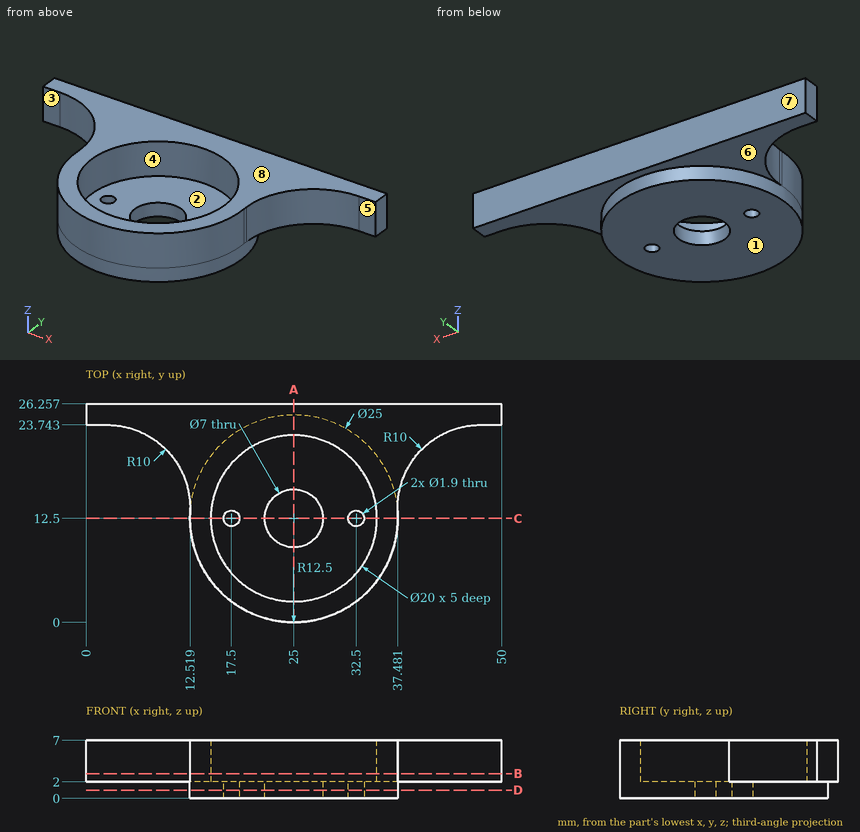
Job drawing, mm, ordinate dimensions from the low corner. One solid piece. A direction names the side the tool comes from. Round coordinates to 2 decimals unless told otherwise and drop trailing zeros. Order: outer loops, then holes, each group sorted by start corner. A loop starts at its lowest first (then second) coordinate and runs counter-clockwise, first axis right, second up. Notation, with made-up numbers: (84.25, -31.5) -> (134.25, -31.5) arc R19 cw to (134.25, -15.5) -> close; hole circle Ø4 at (84, 44.25). An arc over 180 degrees is marked (long way). Write item = value, one per line.
(1) Cut at A-A (x = 25). Write the cut outline in (y, z).
Answers follow:
outline = (0, 0) -> (9, 0) -> (9, 2) -> (2.5, 2) -> (2.5, 7) -> (0, 7) -> close; (16, 0) -> (25, 0) -> (25, 2) -> (26.26, 2) -> (26.26, 7) -> (22.5, 7) -> (22.5, 2) -> (16, 2) -> close
(2) Cut at C-C (y = 12.5). Write the cut outline in (x, z), plus the area to 3 significant figures.
Answers follow:
outline = (12.5, 0) -> (16.55, 0) -> (16.55, 2) -> (15, 2) -> (15, 7) -> (12.5, 7) -> close; (18.45, 0) -> (21.5, 0) -> (21.5, 2) -> (18.45, 2) -> close; (28.5, 0) -> (31.55, 0) -> (31.55, 2) -> (28.5, 2) -> close; (33.45, 0) -> (37.5, 0) -> (37.5, 7) -> (35, 7) -> (35, 2) -> (33.45, 2) -> close
area = 53.4 mm²
(3) Cut at B-B (z = 3). Write the cut outline in (x, y).
Answers follow:
outline = (0, 23.74) -> (2.52, 23.74) arc R10 cw to (12.52, 13.74) -> (12.52, 13.19) arc R12.5 ccw (long way) to (37.48, 13.19) -> (37.48, 13.74) arc R10 cw to (47.48, 23.74) -> (50, 23.74) -> (50, 26.26) -> (0, 26.26) -> close; hole circle Ø20 at (25, 12.5)
(4) Drill centre lines: L1, parallel to Y at x = 32.5, z = 1.4; L2, parallel to Y at x = 25, z = 3.1; L3, parallel to Z at x = 25, y = 5.25. Where is each one in solid material? Low to high.
Answers follow:
L1 = 2.5 to 11.55, 13.45 to 22.5
L2 = 0 to 2.5, 22.5 to 26.26
L3 = 0 to 2
(5) Cut at D-D (z = 1). Write the cut outline in (x, y).
Answers follow:
outline = circle Ø25 at (25, 12.5); hole circle Ø1.9 at (17.5, 12.5); hole circle Ø7 at (25, 12.5); hole circle Ø1.9 at (32.5, 12.5)
(6) Pull direction Y, two halves, no side cores. Call the marked faces 1, 2 and 3: +Y half, -Y half, draft (parallel to the pull), parting line (faces both ways), or undercut.
Answers follow:
face_1 = draft
face_2 = undercut
face_3 = -Y half
(7) 3-axis set-ups, long thin cutter, end or side, ignore diameter. For the marked faces 4, 5, 6, 7 and 8: which of +Z, -Z, +X, -X, +Y, -Y reach the whole face in a straight line?
Answers follow:
face_4 = +Z
face_5 = +Z, -Z, +X, -Y
face_6 = -Z, +Y
face_7 = +Z, -Z, +X, -X, +Y
face_8 = +Z, +X, -X, +Y, -Y
(8) Flat gauge pins, fed straight in: P1, Ø2, axis at x = 12.5, z = 1.5, coming from the -Y side; P2, Ø3, axis at x = 32.5, y = 12.5, coming from the +Z side; P3, Ø2, axis at x = 48, z = 4.5, coming from the -Y side; P4, Ø5.5, axis at x = 25, y = 12.5, coming from the +Z side. Where does each tip first touch, or does it go through?
Answers follow:
P1 = 7.6
P2 = 2
P3 = 23.73
P4 = through
